from build123d import *

# Parameters (mm, degrees)
SKETCH002_R     = 35
PAD001_DEPTH    = 14
SKETCH005_R     = 5.072464
POCKET001_DEPTH = 14
FILLET_R        = 1


with BuildPart() as part:
    # Sketch002 → Pad001 (new body)
    with BuildSketch(Plane.XY.offset(14)):
        Polygon((-31.163938, 31.163938), (-44.072464, 0), (-31.163938, -31.163938), (0, -44.072464), (31.163938, -31.163938), (44.072464, 0), (31.163938, 31.163938), (0, 44.072464), align=None)
        Circle(SKETCH002_R, mode=Mode.SUBTRACT)
    extrude(amount=-PAD001_DEPTH)

    # Sketch005 (on Face10 of Pad001) → Pocket001 (cut)
    with BuildSketch(Plane.XY.offset(14)):
        with Locations((0, 35)):
            Circle(SKETCH005_R)
        with Locations((35, 0)):
            Circle(SKETCH005_R)
        with Locations((0, -35)):
            Circle(SKETCH005_R)
        with Locations((-35, 0)):
            Circle(SKETCH005_R)
    extrude(amount=-POCKET001_DEPTH, mode=Mode.SUBTRACT)

    # Sketch006 → Revolution (revolve)
    with BuildSketch(Plane.XZ):
        Polygon((-40.776272, 0), (-40.043432, 0.680401), (-39.260375, 0), (-35, 0), (-5.289894, -29.463161), (-4.138373, -44.958753), (-5.138373, -44.958753), (-6.25, -30), align=None)
    revolve(axis=Axis((0, 0, 0), (0, 0, 1)))

    # Fillet
    fillet_edges = [part.edges().sort_by_distance(p)[0] for p in [
        (31.163938, 31.163938, 7),
        (15.581969, 37.618201, 14),
        (0, 44.072464, 7),
        (-15.581969, 37.618201, 14),
        (-31.163938, 31.163938, 7),
        (44.072464, 0, 7),
        (37.618201, 15.581969, 14),
        (37.618201, -15.581969, 14),
        (31.163938, -31.163938, 7),
        (15.581969, -37.618201, 14),
        (-15.581969, -37.618201, 14),
        (-37.618201, -15.581969, 14),
        (-37.618201, 15.581969, 14),
        (-44.072464, 0, 7),
        (-31.163938, -31.163938, 7),
        (0, -44.072464, 7),
    ]]
    fillet(fillet_edges, radius=FILLET_R)


solid = part.part
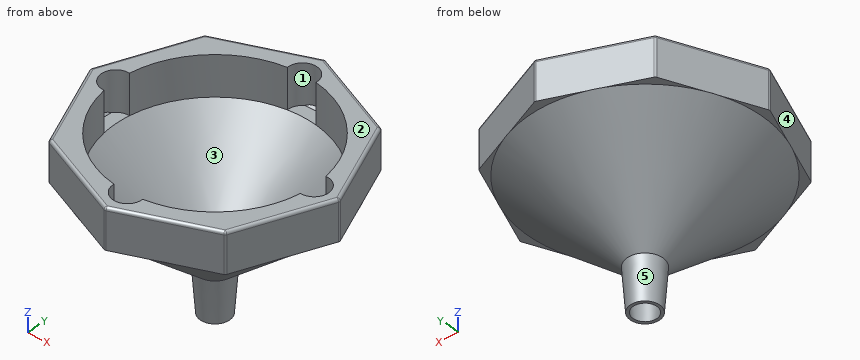
Could you check a few things on this model? Use its own coordinates, in mm. Face numbers are marked on the shaded views. A direction names the side the tool comes from. Coordinates: 2 decimals unless noted, no trailing zeros. Order: outer loops, then holes, each group sorted by start corner. A loop starts at its lowest first (then second) coordinate and runs counter-clockwise, first axis right, second up. Notation, with made-up numbers: (3.25, 61) -> (58.25, 61) arc R10 ccw to (58.25, 75) -> close; hole circle Ø9 at (-1.5, 8). An arc over 180 degrees is marked (long way). One line per item, written item: value. Start each with the question number.
1) Imagine slicing it at B-B on z = -34. List the corners of the cut face in (x, y) for me.
2) Which directions (+Z, -Z, +X, -X, +Y, -Y) give clear straight access to the entire face, cutting with the end or side of a thin tool? Please do the marked faces 1 and 2.
3) We'd pull the mould along X, two halves only. Please class the marked faces 3, 4 and 5: +X half, -X half, draft (parallel to the pull), parting line (faces both ways), or undercut.
4) If I drill on L1, parallel to X at y = 4, z = -21.5 (3 decimals); L2, parallel to Y at x = 28.5, z = 7; L3, parallel to X at y = 3, z = -39, over which ranges is the centre line in solid material (lowest first)? Write a range as [from, to].
5) Imagine slicing it at A-A on z = -40.5. List the corners of the cut face in (x, y) for me.
6) I'm going to push flat-ended pins straight in: pin 1 (3 mm diameter, centred on x = 15, y = -13.5, fed in from +Z); pin 2 (3.5 mm diameter, centred on x = -1, y = 36.5, fed in from +Z); pin 3 (21 mm diameter, centred on x = -30.5, y = 30, fed in from -Z); pin 4 (4 mm diameter, centred on x = -34.5, y = -28.5, fed in from +Z) (3 decimals). Where does each tip first touch, or does it pass through?
Answer list:
1. outline: circle Ø11.91 at (0, 0); hole circle Ø9.91 at (0, 0)
2. face 1: +Z
2. face 2: +Z, +X, -X, +Y, -Y
3. face 3: undercut
3. face 4: -X half
3. face 5: parting line
4. L1: x = [-15.525, -12.705], [12.705, 15.525]
4. L2: y = [-32.27, -20.32], [20.32, 32.27]
4. L3: x = [-4.71, -3.46], [3.46, 4.71]
5. outline: circle Ø10.94 at (0, 0); hole circle Ø8.94 at (0, 0)
6. pin 1: stops at z = -13.21
6. pin 2: stops at z = 0
6. pin 3: stops at z = -7.38
6. pin 4: passes through
